Input: part model. Units: mm. Frame: model coordinates. A direction names the side the tool comes from. Coordinates: 2 decimals unless noted, no trailing zeros. Loops run counter-clockwise (first coordinate to the right, second up) from the corner with the lowest first, then second, coordinate; pieces in that order, holes last. Notation, with made-up numbers: (74, 37.5) - (92, 37.5) arc R23 ccw to (92, 61.5) - close; hole circle Ø6 at (16, -6). An arc over 180 degrees is marked (long way). Use a Markdown table: item, result. Add a question column.
1. Access query for faces 4 (the face through (54.353, -66.972, 4.93)), 5 (the face through (-63.824, -28, 5)). Directions: +Z, -Z, +X, -X, +Y, -Y. A direction counts if a zero-diameter tool reaches every point of the face in a straight line with its end or side. Return the directions, or none.
2. Section query D-D on y = -29. Return the cut outline in (x, z).
3. Draft query along X for faces 1 (the face through (-6, 15.031, 5)), 2 (the face through (-38.824, -28, 5)), 3 (the face through (-67.002, 12.034, 4.93)). Return one class per face: released by +X, released by -X, zero draft, split by the parting line, or undercut.
4. Section query A-A on x = -48. Return the cut outline in (y, z).
5. Section query C-C on z = 6.25. Return the cut outline in (x, y), then the cut area to 3 significant figures.
6. Section query B-B on y = -53. Return the cut outline in (x, z).
7. Ray query, L1, parallel to X at y = -29, z = 7.25; L2, parallel to X at y = -5.5, z = 4; L3, parallel to Y at x = -51, z = 3. Return the intervals inside material, ascending. Write a range as [from, to].
8. Contact query for flat-ended pins moving along their axis: P1, Ø3, axis at x = -55, z = 5.5, coming from the +Y side; P2, Ø1, axis at x = -62.5, z = 9, coming from the +Y side. Output: stop coordinate, or through.
```python
from build123d import *

# Parameters (mm, degrees)
BOSS_EXTRUDE1_DEPTH = 10
SKETCH2_W           = 25
SKETCH2_H           = 65
CUT_EXTRUDE2_DEPTH  = 20
SKETCH3_R           = 10
CUT_EXTRUDE3_DEPTH  = 20


with BuildPart() as part:
    # Sketch1 → Boss-Extrude1 (new body)
    with BuildSketch(Plane.XY):
        with BuildLine():
            Line((-80.798103543, 3.150277686), (-80.798103543, -58.088380877))
            ThreePointArc((-80.798103543, -58.088380877), (-67.213396938, -66.887140682), (-51.324273213, -69.969051596))
            Line((-51.324273213, -69.969051596), (38.675726787, -69.969051596))
            ThreePointArc((38.675726787, -69.969051596), (54.564850513, -66.887140682), (68.149557118, -58.088380877))
            Line((68.149557118, -58.088380877), (68.149557118, 3.150277686))
            ThreePointArc((68.149557118, 3.150277686), (54.564850513, 11.949037491), (38.675726787, 15.030948404))
            Line((38.675726787, 15.030948404), (-51.324273213, 15.030948404))
            ThreePointArc((-51.324273213, 15.030948404), (-67.213396938, 11.949037491), (-80.798103543, 3.150277686))
        make_face()
    extrude(amount=BOSS_EXTRUDE1_DEPTH)

    # Sketch2 → Cut-Extrude2 (cut)
    with BuildSketch(Plane(origin=(0, 0, 0), x_dir=(-1, 0, 0), z_dir=(0, 0, -1))):
        with Locations((51.324273213, -27.469051596)):
            Rectangle(SKETCH2_W, SKETCH2_H)
    extrude(amount=-CUT_EXTRUDE2_DEPTH, mode=Mode.SUBTRACT)

    # Sketch3 → Cut-Extrude3 (cut)
    with BuildSketch(Plane(origin=(0, 0, 0), x_dir=(-1, 0, 0), z_dir=(0, 0, -1))):
        with Locations((-45.543981451, -27.469051596)):
            Circle(SKETCH3_R)
    extrude(amount=-CUT_EXTRUDE3_DEPTH, mode=Mode.SUBTRACT)


solid = part.part
```
Resolved:
| question | item | result |
|---|---|---|
| 1 | face 4 | +Z, -Z, +X, -Y |
| 1 | face 5 | +Z, -Z |
| 2 | outline | (-80.8, 0) - (-63.82, 0) - (-63.82, 10) - (-80.8, 10) - close; (-38.82, 0) - (35.66, 0) - (35.66, 10) - (-38.82, 10) - close; (55.43, 0) - (68.15, 0) - (68.15, 10) - (55.43, 10) - close |
| 3 | face 1 | zero draft |
| 3 | face 2 | undercut |
| 3 | face 3 | released by -X |
| 4 | outline | (-69.97, 0) - (-59.97, 0) - (-59.97, 10) - (-69.97, 10) - close; (5.03, 0) - (15.03, 0) - (15.03, 10) - (5.03, 10) - close |
| 5 | outline | (-80.8, -58.09) arc R42.5 ccw to (-51.32, -69.97) - (38.68, -69.97) arc R42.5 ccw to (68.15, -58.09) - (68.15, 3.15) arc R42.5 ccw to (38.68, 15.03) - (-51.32, 15.03) arc R42.5 ccw to (-80.8, 3.15) - close; hole (-63.82, -59.97) - (-38.82, -59.97) - (-38.82, 5.03) - (-63.82, 5.03) - close; hole circle Ø20 at (45.54, -27.47) |
| 5 | area | 10,300 mm² |
| 6 | outline | (-80.8, 0) - (-63.82, 0) - (-63.82, 10) - (-80.8, 10) - close; (-38.82, 0) - (68.15, 0) - (68.15, 10) - (-38.82, 10) - close |
| 7 | L1 | [-80.8, -63.82], [-38.82, 35.66], [55.43, 68.15] |
| 7 | L2 | [-80.8, -63.82], [-38.82, 68.15] |
| 7 | L3 | [-69.97, -59.97], [5.03, 15.03] |
| 8 | P1 | y = 14.98 |
| 8 | P2 | y = 13.67 |
